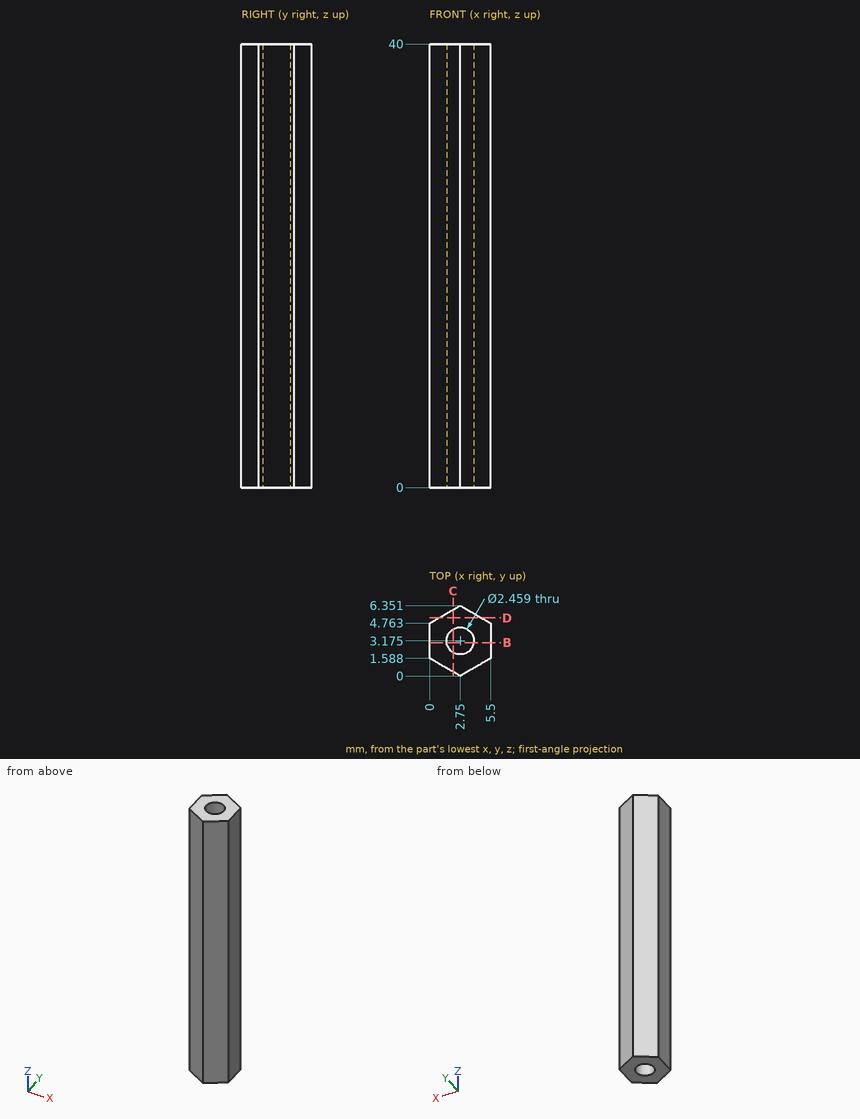
Job drawing, mm, ordinate dimensions from the low corner. One solid piece. Coordinates: 2 decimals unless noted, no trailing zeros. Order: outer loops, then holes, each group sorted by start corner. A loop starts at its lowest first (then second) coordinate and runs counter-clockwise, first axis right, second up. Notation, with made-up numbers: (11, 72.25) -> (70, 72.25) arc R13 cw to (70, 92.25) -> close; hole circle Ø4 at (-18.5, -30.75). An arc over 180 degrees is marked (long way). Answer in a Markdown table with one row per item. Add a question column.
Q1. Band-saw the part on D-D, the plane y = 5.25. List the corners of the cut face in (x, z).
Q2. Wall check: line 1 along X through (y, z) = (3.25, 36.5); line 2 along Y through (x, z) = (2.95, 32.5) (1 decimal); line 3 along X through (y, z) = (3.5, 34) (1 decimal). Give the ranges that are in metal, low to high. Write a range as [from, to].
Q3. Band-saw the part on C-C, the plane x = 2.1. List the corners of the cut face in (y, z) (1 decimal).
Q4. Band-saw the part on B-B, the plane y = 3. List the corners of the cut face in (x, z).
Q5. Drop flat-ended pins along their axis: pin 1 (1.5 mm diameter, centred on x = 1, z = 22.5, fed in from -Y); pin 2 (2 mm diameter, centred on x = 2.75, y = 3.18, fed in from -Z). Give the stop position or say it passes through.
Answers follow:
| question | item | result |
|---|---|---|
| 1 | outline | (0.84, 0) -> (4.66, 0) -> (4.66, 40) -> (0.84, 40) -> close |
| 2 | line 1 | [0, 1.52], [3.98, 5.5] |
| 2 | line 2 | [0.1, 2], [4.4, 6.2] |
| 2 | line 3 | [0, 1.6], [3.9, 5.5] |
| 3 | outline | (0.4, 0) -> (2.1, 0) -> (2.1, 40) -> (0.4, 40) -> close; (4.2, 0) -> (6, 0) -> (6, 40) -> (4.2, 40) -> close |
| 4 | outline | (0, 0) -> (1.53, 0) -> (1.53, 40) -> (0, 40) -> close; (3.97, 0) -> (5.5, 0) -> (5.5, 40) -> (3.97, 40) -> close |
| 5 | pin 1 | y = 0.58 |
| 5 | pin 2 | through |
